Input: part model. Units: mm. Frame: model coordinates. Face numbers are marked on the shaded views. A direction names the side the tool comes from. Coordinates: 2 decimals unless noted, no trailing zeros. Write each loop counter-clockwise with the first axis right and the second up, starting at its lowest first coordinate (ties: lowest second). Pieces come first, ordered by that corner, then holes.
1) Pin query (flat end, axial travel): pin 1 Ø5 at (x, z) = (-24.5, -15.5) entering from +Y; pin 2 Ø1.5 at (y, z) = (-14, 4) entering from +X; pin 3 Ø4 at (y, z) = (-46, 12.5) entering from -X. Return the tip coordinate at first contact, or that it passes through.
2) Draft query along Z for the marked faces 1, 2 and 3. Return one class per face: pulls with the +Z half, pulls with the -Z half, needs draft (parallel to the pull), parting line crosses it, or undercut.
3) Section query A-A (y = -21). Output: boundary loops of the cut face in (x, z) (3 decimals), then the cut area to 3 significant figures.
4) Line query: L1, parallel to Y at x = 13, z = -12.5; L2, parallel to X at y = -21, z = -2.5; L3, parallel to Z at x = 25, y = -7. Output: solid intervals per line, ascending.
5) Set-up query: the marked faces 4 and 5. Return all of +Z, -Z, +X, -X, +Y, -Y with unobstructed straight access to the full face (end or side cutting, diameter ignored); none if empty.
from build123d import *

# Parameters (mm, degrees)
F1_DEPTH = 10.16
F2_R     = 12.7
F3_R     = 12.7
F4_R     = 1.524
F5_R     = 13.97
F6_DEPTH = 43.18
F8_DEPTH = 43.18


with BuildPart() as f1:
    # F0 (on Front) → F1 (new body)
    with BuildSketch(Plane.XZ):
        with BuildLine():
            Line((0, 21.0312), (0, 0))
            Line((0, 0), (21.0312, 0))
            ThreePointArc((21.0312, 0), (25.4, 4.3688), (29.7688, 0))
            Line((29.7688, 0), (42.1132, 0))
            Line((42.1132, 0), (0, 42.1132))
            Line((0, 42.1132), (0, 29.7688))
            ThreePointArc((0, 29.7688), (3.0892081056, 28.4892081056), (4.3688, 25.4))
            ThreePointArc((4.3688, 25.4), (3.0892081056, 22.3107918944), (0, 21.0312))
        make_face()
        with BuildLine():
            Line((21.0312, 0), (0, 0))
            Line((0, 0), (0, -21.0312))
            ThreePointArc((0, -21.0312), (3.0892081056, -22.3107918944), (4.3688, -25.4))
            ThreePointArc((4.3688, -25.4), (3.0892081056, -28.4892081056), (0, -29.7688))
            Line((0, -29.7688), (0, -42.1132))
            Line((0, -42.1132), (42.1132, 0))
            Line((42.1132, 0), (29.7688, 0))
            ThreePointArc((29.7688, 0), (25.4, -4.3688), (21.0312, 0))
        make_face()
        with BuildLine():
            Line((0, -21.0312), (0, 0))
            Line((0, 0), (-21.0312, 0))
            ThreePointArc((-21.0312, 0), (-25.4, -4.3688), (-29.7688, 0))
            Line((-29.7688, 0), (-42.1132, 0))
            Line((-42.1132, 0), (0, -42.1132))
            Line((0, -42.1132), (0, -29.7688))
            ThreePointArc((0, -29.7688), (-4.3688, -25.4), (0, -21.0312))
        make_face()
        with BuildLine():
            Line((-21.0312, 0), (0, 0))
            Line((0, 0), (0, 21.0312))
            ThreePointArc((0, 21.0312), (-4.3688, 25.4), (0, 29.7688))
            Line((0, 29.7688), (0, 42.1132))
            Line((0, 42.1132), (-42.1132, 0))
            Line((-42.1132, 0), (-29.7688, 0))
            ThreePointArc((-29.7688, 0), (-25.4, 4.3688), (-21.0312, 0))
        make_face()
    extrude(amount=F1_DEPTH)

    # F2
    f2_edges = [f1.edges().sort_by_distance(p)[0] for p in [
        (0, -5.08, 42.1132),
        (-42.1132, -5.08, 0),
    ]]
    fillet(f2_edges, radius=F2_R)

    # F3
    f3_edges = [f1.edges().sort_by_distance(p)[0] for p in [
        (42.1132, -5.08, 0),
        (0, -5.08, -42.1132),
    ]]
    fillet(f3_edges, radius=F3_R)

    # F4
    f4_edges = [f1.edges().sort_by_distance(p)[0] for p in [
        (-21.0566, -10.16, 21.0566),
        (0, -10.16, 36.852688),
        (21.0566, -10.16, 21.0566),
        (36.852688, -10.16, 0),
        (21.0566, -10.16, -21.0566),
        (0, -10.16, -36.852688),
        (-21.0566, -10.16, -21.0566),
        (-36.852688, -10.16, 0),
    ]]
    fillet(f4_edges, radius=F4_R)

    # F5 (on face) → F6 (join)
    with BuildSketch(Plane.XZ.offset(10.16)):
        Circle(F5_R)
    extrude(amount=F6_DEPTH)

    # F7 (on face) → F8 (cut)
    with BuildSketch(Plane.XZ.offset(53.34)):
        with BuildLine():
            Line((0, 0), (9.525, 0))
            ThreePointArc((9.525, 0), (6.7351920908, 6.7351920908), (0, 9.525))
            Line((0, 9.525), (0, 0))
        make_face()
        with BuildLine():
            Line((0, 0), (0, 9.525))
            ThreePointArc((0, 9.525), (-6.7351920908, 6.7351920908), (-9.525, 0))
            Line((-9.525, 0), (0, 0))
        make_face()
        with BuildLine():
            ThreePointArc((-9.525, 0), (-6.7351920908, -6.7351920908), (0, -9.525))
            Line((0, -9.525), (0, 0))
            Line((0, 0), (-9.525, 0))
        make_face()
        with BuildLine():
            ThreePointArc((0, -9.525), (6.7351920908, -6.7351920908), (9.525, 0))
            Line((9.525, 0), (0, 0))
            Line((0, 0), (0, -9.525))
        make_face()
    extrude(amount=-F8_DEPTH, mode=Mode.SUBTRACT)


solid = f1.part
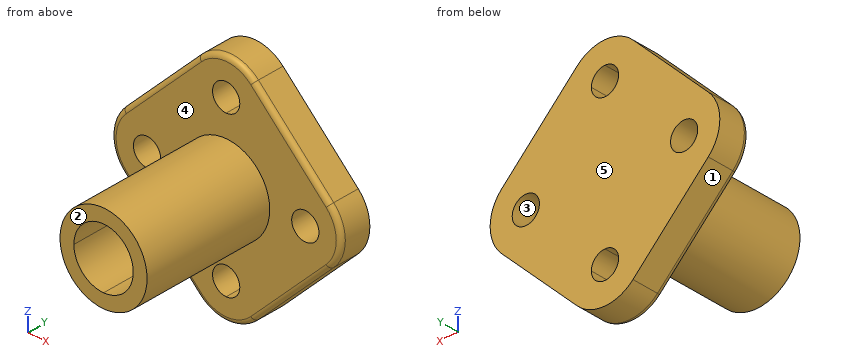
Answer:
1. pin 1: stops at y = 0
1. pin 2: stops at x = 13.59
1. pin 3: stops at x = -9.21
2. face 1: pulls with the -Z half
2. face 2: needs draft
2. face 3: undercut
3. outline: circle Ø27.94 at (0, 0); hole circle Ø19.05 at (0, 0)
3. area: 328 mm2
4. L1: y = -10.16 to 0
4. L2: x = -13.74 to -9.19, 9.19 to 13.74
4. L3: z = -17.11 to -4.35, 4.35 to 17.11
5. face 4: -Y
5. face 5: +Z, -Z, +X, -X, +Y
